Verification items for this drawing (mm, ordinates from the low corner). A direction names the side the tool comes from. Round coordinates to 2 decimals unless told otherwise and drop trailing zeros. Write each loop counter-clockwise with the first axis right and the second up, starting at its lowest first coordinate (ties: lowest second). Pieces come first, ordered by that corner, then holes. Notation, with made-up numbers: M 3,87.25 L 26,87.25 A15 cw 26,96.25 Z; hole C 40.25,40 d2. An arc over 180 degrees is marked long. Write each question's results on one line, items separated by ' | '.
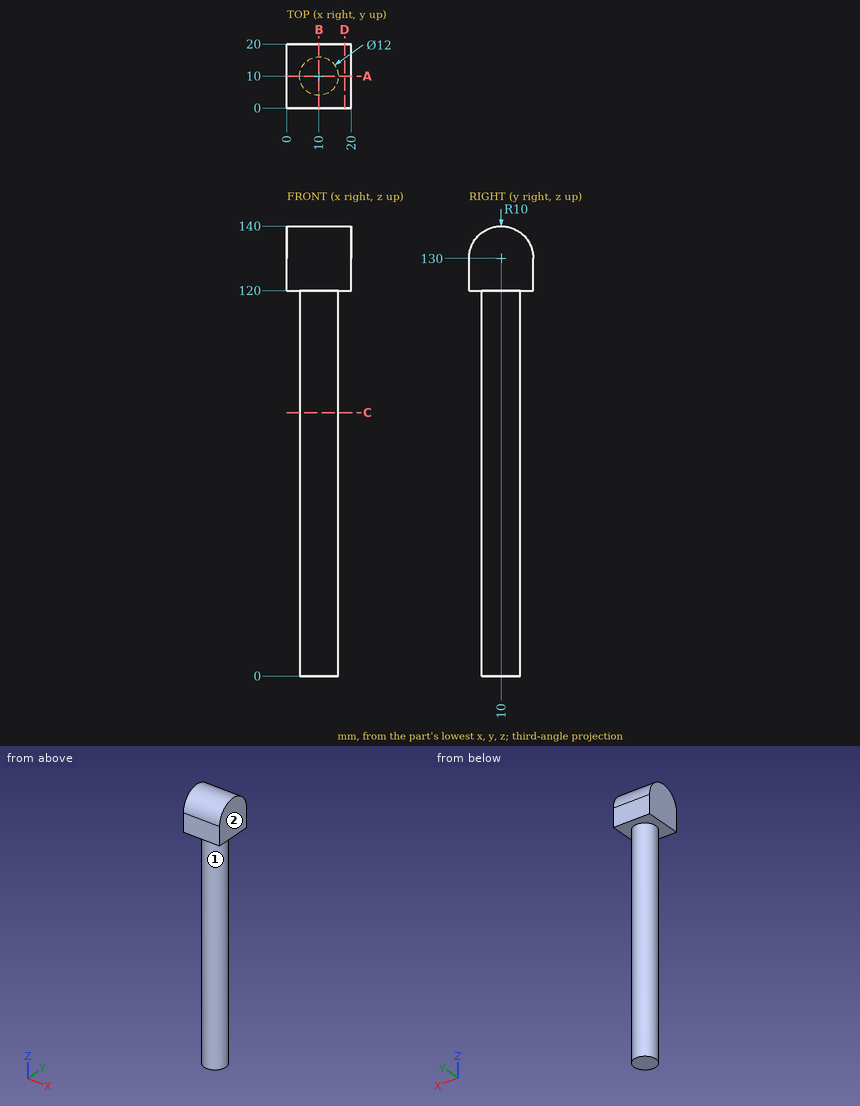
1) Sectioned sample at B-B, the plane x = 10. Record the cut outline in (y, z), and give its area (3 significant figures).
Calculated:
outline: M 0,120 L 4,120 L 4,0 L 16,0 L 16,120 L 20,120 L 20,130 A10 ccw 0,130 Z | area: 1,800 mm²
2) Depth check by flat-ended pin: P1, Ø2, axis at x = 9, z = 41, coming from the +Y side; P2, Ø1, axis at x = 5.5, y = 8, coming from the +Z side; P3, Ø8, axis at y = 3.5, z = 38.5, coming from the -X side. Enter the tip coordinate at first touch or a pass-through.
Calculated:
P1: stops at y = 16 | P2: stops at z = 139.89 | P3: stops at x = 4.55
3) Material ranges on line 1 (Y direction, x = 9.5, z = 68); line 2 (X direction, y = 9.75, z = 29); line 3 (X direction, y = 5.75, z = 84.5), recorded low to high. Write a range as [from, to].
Calculated:
line 1: y = [4.02, 15.98] | line 2: x = [4.01, 15.99] | line 3: x = [5.76, 14.24]
4) Access from +Z, -Z, +X, -X, +Y, -Y to the whole of each face (thin tool, end or side, straight path). Record for the marked faces 1 and 2.
Calculated:
face 1: -Z | face 2: +Z, -Z, +X, +Y, -Y
5) Sectioned sample at A-A, the plane y = 10. Record the cut outline in (x, z), and give its area (3 significant figures).
Calculated:
outline: M 0,120 L 4,120 L 4,0 L 16,0 L 16,120 L 20,120 L 20,140 L 0,140 Z | area: 1,840 mm²
6) Sectioned sample at C-C, the plane z = 82. Record the cut outline in (x, y), and give its area (3 significant figures).
Calculated:
outline: C 10,10 d12 | area: 113 mm²
7) Sectioned sample at D-D, the plane x = 18. Record the cut outline in (y, z), and give its area (3 significant figures).
Calculated:
outline: M 0,120 L 20,120 L 20,130 A10 ccw 0,130 Z | area: 357 mm²
